Design review of the part built by this model. Coordinates are the model's own, in mm. A direction names the side the tool comes from. Coordinates: 2 decimals unless noted, no trailing zeros. Answer as a JSON object with one key per item and string values.
```python
from build123d import *

# Parameters (mm, degrees)
EXTRUDE1_DEPTH = 300


with BuildPart() as part:
    # Sketch1 → Extrude1 (new body)
    with BuildSketch(Plane.XY):
        with BuildLine():
            Line((-5.032287798, -0.341059771), (-5.516287798, -0.341059771))
            ThreePointArc((-5.516287798, -0.341059771), (-5.875498042, -0.192270016), (-6.024287798, 0.166940229))
            Line((-6.024287798, 0.166940229), (-6.024287798, 2.515940229))
            ThreePointArc((-6.024287798, 2.515940229), (-6.173077553, 2.875150474), (-6.532287798, 3.023940229))
            Line((-6.532287798, 3.023940229), (-7.258207136, 3.023940229))
            ThreePointArc((-7.258207136, 3.023940229), (-7.45261032, 2.985271032), (-7.617417381, 2.875150474))
            Line((-7.617417381, 2.875150474), (-10.720498042, -0.227930187))
            ThreePointArc((-10.720498042, -0.227930187), (-10.8306186, -0.392737249), (-10.869287798, -0.587140432))
            Line((-10.869287798, -0.587140432), (-10.869287798, -5.354979109))
            ThreePointArc((-10.869287798, -5.354979109), (-10.8306186, -5.549382293), (-10.720498042, -5.714189354))
            Line((-10.720498042, -5.714189354), (-7.617417381, -8.817270016))
            ThreePointArc((-7.617417381, -8.817270016), (-7.45261032, -8.927390573), (-7.258207136, -8.966059771))
            Line((-7.258207136, -8.966059771), (-6.532287798, -8.966059771))
            ThreePointArc((-6.532287798, -8.966059771), (-6.173077553, -8.817270016), (-6.024287798, -8.458059771))
            Line((-6.024287798, -8.458059771), (-6.024287798, -6.109059771))
            ThreePointArc((-6.024287798, -6.109059771), (-5.875498042, -5.749849526), (-5.516287798, -5.601059771))
            Line((-5.516287798, -5.601059771), (-5.032287798, -5.601059771))
            ThreePointArc((-5.032287798, -5.601059771), (-4.673077553, -5.749849526), (-4.524287798, -6.109059771))
            Line((-4.524287798, -6.109059771), (-4.524287798, -11.471059771))
            ThreePointArc((-4.524287798, -11.471059771), (-4.963627626, -12.531719943), (-6.024287798, -12.971059771))
            Line((-6.024287798, -12.971059771), (-11.386287798, -12.971059771))
            ThreePointArc((-11.386287798, -12.971059771), (-11.745498042, -12.822270016), (-11.894287798, -12.463059771))
            Line((-11.894287798, -12.463059771), (-11.894287798, -11.979059771))
            ThreePointArc((-11.894287798, -11.979059771), (-11.745498042, -11.619849526), (-11.386287798, -11.471059771))
            Line((-11.386287798, -11.471059771), (-9.037287798, -11.471059771))
            ThreePointArc((-9.037287798, -11.471059771), (-8.678077553, -11.322270016), (-8.529287798, -10.963059771))
            Line((-8.529287798, -10.963059771), (-8.529287798, -10.237140432))
            ThreePointArc((-8.529287798, -10.237140432), (-8.567956995, -10.042737249), (-8.678077553, -9.877930187))
            Line((-8.678077553, -9.877930187), (-11.781158214, -6.774849526))
            ThreePointArc((-11.781158214, -6.774849526), (-11.945965275, -6.664728968), (-12.140368459, -6.626059771))
            Line((-12.140368459, -6.626059771), (-16.908207136, -6.626059771))
            ThreePointArc((-16.908207136, -6.626059771), (-17.10261032, -6.664728968), (-17.267417381, -6.774849526))
            Line((-17.267417381, -6.774849526), (-20.370498042, -9.877930187))
            ThreePointArc((-20.370498042, -9.877930187), (-20.4806186, -10.042737249), (-20.519287798, -10.237140432))
            Line((-20.519287798, -10.237140432), (-20.519287798, -10.963059771))
            ThreePointArc((-20.519287798, -10.963059771), (-20.370498042, -11.322270016), (-20.011287798, -11.471059771))
            Line((-20.011287798, -11.471059771), (-17.662287798, -11.471059771))
            ThreePointArc((-17.662287798, -11.471059771), (-17.303077553, -11.619849526), (-17.154287798, -11.979059771))
            Line((-17.154287798, -11.979059771), (-17.154287798, -12.463059771))
            ThreePointArc((-17.154287798, -12.463059771), (-17.303077553, -12.822270016), (-17.662287798, -12.971059771))
            Line((-17.662287798, -12.971059771), (-23.024287798, -12.971059771))
            ThreePointArc((-23.024287798, -12.971059771), (-24.084947969, -12.531719943), (-24.524287798, -11.471059771))
            Line((-24.524287798, -11.471059771), (-24.524287798, -6.109059771))
            ThreePointArc((-24.524287798, -6.109059771), (-24.375498042, -5.749849526), (-24.016287798, -5.601059771))
            Line((-24.016287798, -5.601059771), (-23.532287798, -5.601059771))
            ThreePointArc((-23.532287798, -5.601059771), (-23.173077553, -5.749849526), (-23.024287798, -6.109059771))
            Line((-23.024287798, -6.109059771), (-23.024287798, -8.458059771))
            ThreePointArc((-23.024287798, -8.458059771), (-22.875498042, -8.817270016), (-22.516287798, -8.966059771))
            Line((-22.516287798, -8.966059771), (-21.790368459, -8.966059771))
            ThreePointArc((-21.790368459, -8.966059771), (-21.595965275, -8.927390573), (-21.431158214, -8.817270016))
            Line((-21.431158214, -8.817270016), (-18.328077553, -5.714189354))
            ThreePointArc((-18.328077553, -5.714189354), (-18.217956995, -5.549382293), (-18.179287798, -5.354979109))
            Line((-18.179287798, -5.354979109), (-18.179287798, -0.587140432))
            ThreePointArc((-18.179287798, -0.587140432), (-18.217956995, -0.392737249), (-18.328077553, -0.227930187))
            Line((-18.328077553, -0.227930187), (-21.431158214, 2.875150474))
            ThreePointArc((-21.431158214, 2.875150474), (-21.595965275, 2.985271032), (-21.790368459, 3.023940229))
            Line((-21.790368459, 3.023940229), (-22.516287798, 3.023940229))
            ThreePointArc((-22.516287798, 3.023940229), (-22.875498042, 2.875150474), (-23.024287798, 2.515940229))
            Line((-23.024287798, 2.515940229), (-23.024287798, 0.166940229))
            ThreePointArc((-23.024287798, 0.166940229), (-23.173077553, -0.192270016), (-23.532287798, -0.341059771))
            Line((-23.532287798, -0.341059771), (-24.016287798, -0.341059771))
            ThreePointArc((-24.016287798, -0.341059771), (-24.375498042, -0.192270016), (-24.524287798, 0.166940229))
            Line((-24.524287798, 0.166940229), (-24.524287798, 5.528940229))
            ThreePointArc((-24.524287798, 5.528940229), (-24.084947969, 6.589600401), (-23.024287798, 7.028940229))
            Line((-23.024287798, 7.028940229), (-17.662287798, 7.028940229))
            ThreePointArc((-17.662287798, 7.028940229), (-17.303077553, 6.880150474), (-17.154287798, 6.520940229))
            Line((-17.154287798, 6.520940229), (-17.154287798, 6.036940229))
            ThreePointArc((-17.154287798, 6.036940229), (-17.303077553, 5.677729984), (-17.662287798, 5.528940229))
            Line((-17.662287798, 5.528940229), (-20.011287798, 5.528940229))
            ThreePointArc((-20.011287798, 5.528940229), (-20.370498042, 5.380150474), (-20.519287798, 5.020940229))
            Line((-20.519287798, 5.020940229), (-20.519287798, 4.295020891))
            ThreePointArc((-20.519287798, 4.295020891), (-20.4806186, 4.100617707), (-20.370498042, 3.935810646))
            Line((-20.370498042, 3.935810646), (-17.267417381, 0.832729984))
            ThreePointArc((-17.267417381, 0.832729984), (-17.10261032, 0.722609427), (-16.908207136, 0.683940229))
            Line((-16.908207136, 0.683940229), (-12.140368459, 0.683940229))
            ThreePointArc((-12.140368459, 0.683940229), (-11.945965275, 0.722609427), (-11.781158214, 0.832729984))
            Line((-11.781158214, 0.832729984), (-8.678077553, 3.935810646))
            ThreePointArc((-8.678077553, 3.935810646), (-8.567956995, 4.100617707), (-8.529287798, 4.295020891))
            Line((-8.529287798, 4.295020891), (-8.529287798, 5.020940229))
            ThreePointArc((-8.529287798, 5.020940229), (-8.678077553, 5.380150474), (-9.037287798, 5.528940229))
            Line((-9.037287798, 5.528940229), (-11.386287798, 5.528940229))
            ThreePointArc((-11.386287798, 5.528940229), (-11.745498042, 5.677729984), (-11.894287798, 6.036940229))
            Line((-11.894287798, 6.036940229), (-11.894287798, 6.520940229))
            ThreePointArc((-11.894287798, 6.520940229), (-11.745498042, 6.880150474), (-11.386287798, 7.028940229))
            Line((-11.386287798, 7.028940229), (-6.024287798, 7.028940229))
            ThreePointArc((-6.024287798, 7.028940229), (-4.963627626, 6.589600401), (-4.524287798, 5.528940229))
            Line((-4.524287798, 5.528940229), (-4.524287798, 0.166940229))
            ThreePointArc((-4.524287798, 0.166940229), (-4.673077553, -0.192270016), (-5.032287798, -0.341059771))
        make_face()
        with BuildLine():
            Line((-12.399386954, -5.275565737), (-12.219781831, -5.095960615))
            ThreePointArc((-12.219781831, -5.095960615), (-12.018349781, -4.327527582), (-12.589154291, -3.775036489))
            ThreePointArc((-12.589154291, -3.775036489), (-12.428787798, -2.971059771), (-12.589154291, -2.167083053))
            ThreePointArc((-12.589154291, -2.167083053), (-12.018349781, -1.61459196), (-12.219781831, -0.846158927))
            Line((-12.219781831, -0.846158927), (-12.399386954, -0.666553805))
            ThreePointArc((-12.399386954, -0.666553805), (-13.167819987, -0.465121754), (-13.72031108, -1.035926265))
            ThreePointArc((-13.72031108, -1.035926265), (-14.524287798, -0.875559771), (-15.328264516, -1.035926265))
            ThreePointArc((-15.328264516, -1.035926265), (-15.880755608, -0.465121754), (-16.649188641, -0.666553805))
            Line((-16.649188641, -0.666553805), (-16.828793764, -0.846158927))
            ThreePointArc((-16.828793764, -0.846158927), (-17.030225814, -1.61459196), (-16.459421304, -2.167083053))
            ThreePointArc((-16.459421304, -2.167083053), (-16.619787798, -2.971059771), (-16.459421304, -3.775036489))
            ThreePointArc((-16.459421304, -3.775036489), (-17.030225814, -4.327527582), (-16.828793764, -5.095960615))
            Line((-16.828793764, -5.095960615), (-16.649188641, -5.275565737))
            ThreePointArc((-16.649188641, -5.275565737), (-15.880755608, -5.476997788), (-15.328264516, -4.906193277))
            ThreePointArc((-15.328264516, -4.906193277), (-14.524287798, -5.066559771), (-13.72031108, -4.906193277))
            ThreePointArc((-13.72031108, -4.906193277), (-13.167819987, -5.476997788), (-12.399386954, -5.275565737))
        make_face(mode=Mode.SUBTRACT)
    extrude(amount=EXTRUDE1_DEPTH)


solid = part.part
```
1) Clearance check with a flat-ended pin moving along its axis: pin 1 Ø2.5 at (y, z) = (-4, 221) entering from -X. State where the tip first meets the part, or that it passes through.
Completed:
{"pin 1": "x = -18.18"}
2) The part is to be moulded in two halves that separate along Y. For faces 1 (the flat face through (-10.869, -3, 148)), 2 (the flat face through (-14, -6.626, 148)), 3 (the flat face through (-18.179, -3, 148)), 4 (the flat face through (-20, 7.029, 148)), say which applies: pulls with the +Y half, pulls with the -Y half, needs draft (parallel to the pull), parting line crosses it, or undercut.
Completed:
{"face 1": "undercut", "face 2": "pulls with the -Y half", "face 3": "undercut", "face 4": "pulls with the +Y half"}
3) Wall thickness on probe 1 along Y at (x, z) = (-7.5, 85.5); probe 2 along X at (y, z) = (-5.75, 166); probe 3 along Y at (x, z) = (-18.25, 158.5): over which ranges is each line inside the solid? List them lowest first.
Completed:
{"probe 1": "-12.97 to -8.9, 2.96 to 7.03", "probe 2": "-24.38 to -23.17, -18.36 to -10.68, -5.88 to -4.67", "probe 3": "-12.97 to -11.47, -7.76 to -5.61, -0.33 to 1.82, 5.53 to 7.03"}
4) For faces 5 (the flat face through (-15, 0.684, 148)), 6 (the flat face through (-9, 7.029, 148)), list the 3-axis set-ups (+Z, -Z, +X, -X, +Y, -Y) from which the entire face can be reached by the end or side of a thin tool; tool diameter is ignored.
Completed:
{"face 5": "+Z, -Z, +Y", "face 6": "+Z, -Z, +X, -X, +Y"}
